Part model, mm, in its own coordinate system. Give positions to 0.01 mm unless a question says otherwise; leave off trailing zeros. Order: outer loops, then holes, each group sorted by start corner. A loop starts at its lowest first (then second) coordinate and runs counter-clockwise, first axis right, second up. Notation, with made-up numbers: (-23.5, -28) - (15.5, -28) arc R16 cw to (15.5, -1) - close; hole circle Ø9 at (50.25, 30). An arc over 180 degrees is marked (long way). Use a Markdown table: item, result. Add a question column.
from build123d import *

# Parameters (mm, degrees)
SKETCH1_W                      = 90
SKETCH1_H                      = 30
BOSS_EXTRUDE1_DEPTH            = 1.5
M5_CLEARANCE_HOLE1_D           = 5.5
M5_CLEARANCE_HOLE1_CSINK_D     = 5.55
M5_CLEARANCE_HOLE1_CSINK_ANGLE = 90


with BuildPart() as part:
    # Sketch1 → Boss-Extrude1 (new, symmetric)
    with BuildSketch(Plane.XY):
        Rectangle(SKETCH1_W, SKETCH1_H)
    extrude(amount=BOSS_EXTRUDE1_DEPTH, both=True)

    # M5 Clearance Hole1 (through all)
    with Locations(Plane.XY.offset(1.5)):
        with Locations((12.5, 4.5), (-12.5, 4.5)):
            CounterSinkHole(M5_CLEARANCE_HOLE1_D / 2, M5_CLEARANCE_HOLE1_CSINK_D / 2, counter_sink_angle=M5_CLEARANCE_HOLE1_CSINK_ANGLE)


solid = part.part
1. Cut at B-B (x = -12.5). Write the cut outline in (y, z) (3 decimals).
2. Cut at A-A (y = 4.5). Write the cut outline in (x, z) (3 decimals), plus the area to 3 significant figures.
3. Drill centre lines: probe 1 along X at (y, z) = (4.5, -0.25); probe 2 along Y at (x, z) = (-12.5, -0.6); probe 3 along X at (y, z) = (5.5, 0). Where is each one in solid material? Low to high. Write a range as [from, to].
4. Mould opens along Y. For faces 1 (the face through (-13.77, 2.06, -0.03)), 2 (the face through (45, 0, 0)), 3 (the face through (-1, -15, 0)) say: released by +Y, released by -Y, zero draft, split by the parting line, or undercut.
5. Cut at C-C (z = -0.6). Write the cut outline in (x, y).
Responses:
| question | item | result |
|---|---|---|
| 1 | outline | (-15, -1.5) - (1.75, -1.5) - (1.75, 1.475) - (1.725, 1.5) - (-15, 1.5) - close; (7.25, -1.5) - (15, -1.5) - (15, 1.5) - (7.275, 1.5) - (7.25, 1.475) - close |
| 2 | outline | (-45, -1.5) - (-15.25, -1.5) - (-15.25, 1.475) - (-15.275, 1.5) - (-45, 1.5) - close; (-9.75, -1.5) - (9.75, -1.5) - (9.75, 1.475) - (9.725, 1.5) - (-9.725, 1.5) - (-9.75, 1.475) - close; (15.25, -1.5) - (45, -1.5) - (45, 1.5) - (15.275, 1.5) - (15.25, 1.475) - close |
| 2 | area | 237 mm² |
| 3 | probe 1 | x = [-45, -15.25], [-9.75, 9.75], [15.25, 45] |
| 3 | probe 2 | y = [-15, 1.75], [7.25, 15] |
| 3 | probe 3 | x = [-45, -15.06], [-9.94, 9.94], [15.06, 45] |
| 4 | face 1 | undercut |
| 4 | face 2 | zero draft |
| 4 | face 3 | released by -Y |
| 5 | outline | (-45, -15) - (45, -15) - (45, 15) - (-45, 15) - close; hole circle Ø5.5 at (-12.5, 4.5); hole circle Ø5.5 at (12.5, 4.5) |
